CAD build for the part. Positions are in the model's coordinates, mm. A direction names the side the tool comes from. Coordinates: 2 decimals unless noted, no trailing zeros. Write each loop counter-clockwise with the first axis right and the second up, starting at its lowest first coordinate (ties: lowest second). Pieces come first, ordered by that corner, then holes. Notation, with made-up numbers: (-33, 19) - (3, 19) arc R23 cw to (3, 56) - close; hole circle Ø10 at (62.25, 84.25). An arc over 180 degrees is marked (long way). Answer in a Markdown table with one row per item. Add a question column.
Q1. Band-saw the part on C-C (x = 0). List the corners of the cut face in (y, z), and give its area (3 significant figures).
Q2. Two-plate mould, pull along X, no slides. Class faces 5 (the cylindrical face through (-0.976, -12.064, 1.521)), 6 (the flat face through (-41, 29, 1)), 7 (the flat face through (-29, 39.5, 1)): +X half, -X half, draft (parallel to the pull), parting line (faces both ways), or undercut.
Q3. Pin check, flat tips, straight feed: pin 1 (12 mm diameter, centred on x = 0, y = -19.5, fed in from +Z); pin 2 (0.9 mm diameter, centred on x = -29, z = 1.5, fed in from +Y); pin 3 (0.9 mm diameter, centred on x = 39, z = 1.5, fed in from +Y); pin 4 (0.9 mm diameter, centred on y = -32.5, z = 2, fed in from +X). Stop position of each tip, or through.
Q4. Band-saw the part on B-B (z = 2.25). List the corners of the cut face in (x, y).
Q5. Drill centre lines: line 1 along Y through (x, z) = (0, 1.45); line 2 along X through (y, z) = (-9.5, 2.6); line 3 along X through (y, z) = (-27.5, 2). Where is each one in solid material? Low to high. Write a range as from..to.
Q6. Band-saw the part on A-A (y = -19.5). List the corners of the cut face in (x, z).
Q7. Band-saw the part on D-D (x = 24.5). List the corners of the cut face in (y, z), and give its area (3 significant figures).
Q8. 3-axis set-ups, long thin cutter, end or side, ignore diameter. For faces 1 (the flat face through (-17.5, 41, 1)), 2 (the flat face through (17.5, 41, 1)), 3 (the flat face through (38, -28, 1)), 4 (the flat face through (-38, 2, 1)): which of +Z, -Z, +X, -X, +Y, -Y reach the whole face in a straight line?
```python
from build123d import *

# Parameters (mm, degrees)
BOSS_EXTRUDE1_DEPTH = 3
SKETCH2_R           = 7.5
CUT_EXTRUDE1_DEPTH  = 3


with BuildPart() as part:
    # Sketch1 → Boss-Extrude1 (new body)
    with BuildSketch(Plane.XY):
        Polygon((-38, 39.5), (-17.5, 39.5), (-17.5, 42.5), (17.5, 42.5), (17.5, 39.5), (38, 39.5), (38, 19), (41, 19), (41, 16), (41, -16), (38, -16), (38, -19), (38, -39.5), (-41, -39.5), (-41, -19), (-41, -16), (-38, -16), (-38, 16), (-38, 19), (-41, 19), (-41, 39.5), align=None)
    extrude(amount=BOSS_EXTRUDE1_DEPTH)

    # Sketch2 → Cut-Extrude1 (cut)
    with BuildSketch(Plane.XY.offset(3)):
        with Locations((0, -19.5)):
            Circle(SKETCH2_R)
    extrude(amount=-CUT_EXTRUDE1_DEPTH, mode=Mode.SUBTRACT)


solid = part.part
```
Checked values:
| question | item | result |
|---|---|---|
| 1 | outline | (-39.5, 0) - (-27, 0) - (-27, 3) - (-39.5, 3) - close; (-12, 0) - (42.5, 0) - (42.5, 3) - (-12, 3) - close |
| 1 | area | 201 mm² |
| 2 | face 5 | undercut |
| 2 | face 6 | -X half |
| 2 | face 7 | draft |
| 3 | pin 1 | passes through |
| 3 | pin 2 | stops at y = 39.5 |
| 3 | pin 3 | stops at y = 19 |
| 3 | pin 4 | stops at x = 38 |
| 4 | outline | (-41, -39.5) - (38, -39.5) - (38, -16) - (41, -16) - (41, 19) - (38, 19) - (38, 39.5) - (17.5, 39.5) - (17.5, 42.5) - (-17.5, 42.5) - (-17.5, 39.5) - (-41, 39.5) - (-41, 19) - (-38, 19) - (-38, -16) - (-41, -16) - close; hole circle Ø15 at (0, -19.5) |
| 5 | line 1 | y = -39.5..-27, -12..42.5 |
| 5 | line 2 | x = -38..41 |
| 5 | line 3 | x = -41..38 |
| 6 | outline | (-41, 0) - (-7.5, 0) - (-7.5, 3) - (-41, 3) - close; (7.5, 0) - (38, 0) - (38, 3) - (7.5, 3) - close |
| 7 | outline | (-39.5, 0) - (39.5, 0) - (39.5, 3) - (-39.5, 3) - close |
| 7 | area | 237 mm² |
| 8 | face 1 | +Z, -Z, -X, +Y |
| 8 | face 2 | +Z, -Z, +X, +Y |
| 8 | face 3 | +Z, -Z, +X, -Y |
| 8 | face 4 | +Z, -Z, -X |
